Can you work these out from the model? Positions are in its coordinate system, mm. Face numbers are marked on the shaded views. A direction names the side the tool comes from. Round coordinates to 2 decimals unless told otherwise and drop trailing zeros. Loops run counter-clockwise (first coordinate to the right, second up) from the corner with the lowest first, then second, coordinate; pieces in that order, holes last. Notation, with made-up numbers: M -24.5,24.25 L 26.5,24.25 A6 cw 26.5,32.25 Z; hole C 49.25,-27 d6. An arc over 180 degrees is marked long. Answer as CSV lines item,"result".
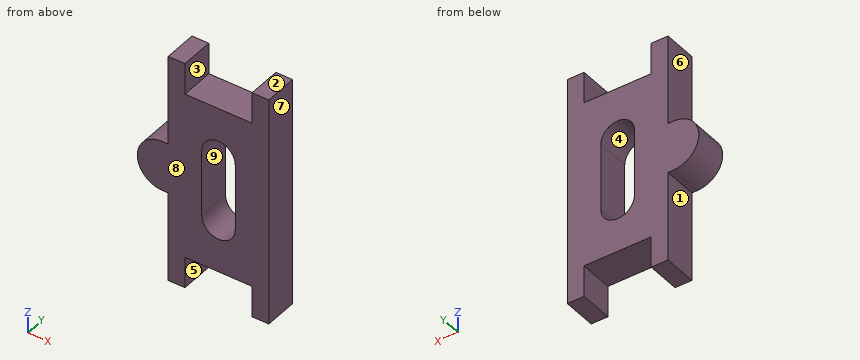
from build123d import *

# Parameters (mm, degrees)
BOSS_EXTRUDE1_DEPTH = 3.175
CUT_EXTRUDE1_REACH  = 5.175


with BuildPart() as part:
    # Sketch2 → Boss-Extrude1 (new body)
    with BuildSketch(Plane(origin=(0, 0, 0), x_dir=(1, 0, 0), z_dir=(0, 1, 0))):
        with BuildLine():
            Line((-3.175, 10.8966), (-3.175, 7.9375))
            Line((-3.175, 7.9375), (3.175, 7.9375))
            Line((3.175, 7.9375), (3.175, 10.8966))
            Line((3.175, 10.8966), (4.7625, 10.8966))
            Line((4.7625, 10.8966), (4.7625, -10.8966))
            Line((4.7625, -10.8966), (3.175, -10.8966))
            Line((3.175, -10.8966), (3.175, -7.9375))
            Line((3.175, -7.9375), (-3.175, -7.9375))
            Line((-3.175, -7.9375), (-3.175, -10.8966))
            Line((-3.175, -10.8966), (-4.7625, -10.8966))
            Line((-4.7625, -10.8966), (-4.7625, -2.38125))
            Line((-4.7625, -2.38125), (-5.30225, -2.38125))
            ThreePointArc((-5.30225, -2.38125), (-7.6835, 0), (-5.30225, 2.38125))
            Line((-5.30225, 2.38125), (-4.7625, 2.38125))
            Line((-4.7625, 2.38125), (-4.7625, 10.8966))
            Line((-4.7625, 10.8966), (-3.175, 10.8966))
        make_face()
    extrude(amount=BOSS_EXTRUDE1_DEPTH)

    # Sketch3 → Cut-Extrude1 (cut, up to next)
    with BuildSketch(Plane(origin=(0, 3.175, 0), x_dir=(1, 0, 0), z_dir=(0, 1, 0)), mode=Mode.PRIVATE) as cut_extrude1_sk1:
        with BuildLine():
            Line((1.5875, 3.175), (1.5875, -3.175))
            ThreePointArc((1.5875, -3.175), (0, -4.7625), (-1.5875, -3.175))
            Line((-1.5875, -3.175), (-1.5875, 3.175))
            ThreePointArc((-1.5875, 3.175), (0, 4.7625), (1.5875, 3.175))
        make_face()
    cut_extrude1_tool1 = extrude(cut_extrude1_sk1.sketch, amount=-CUT_EXTRUDE1_REACH, mode=Mode.PRIVATE) & part.part
    add(cut_extrude1_tool1.solids().sort_by_distance((0, 3.175, 0))[0], mode=Mode.SUBTRACT)


solid = part.part
Item 1: If I drill on line 1 along X through (y, z) = (0.65, 10.25) (1 decimal); line 2 along X through (y, z) = (2.8, -2.5); line 3 along X through (y, z) = (0.75, -5.75), over which ranges is the centre line in solid material (lowest first)? Write a range as from..to.
Output:
line 1,"x = -4.8..-3.2, 3.2..4.8"
line 2,"x = -4.76..-1.59, 1.59..4.76"
line 3,"x = -4.76..4.76"
Item 2: If we section it at C-C on x = 0: Write out the boundary of the cut face in (y, z) (1 decimal).
Output:
outline,"M 0,-7.9 L 3.2,-7.9 L 3.2,-4.8 L 0,-4.8 Z; M 0,4.8 L 3.2,4.8 L 3.2,7.9 L 0,7.9 Z"
Item 3: On a 3-axis mill with a long thin cutter (end or side, diameter ignored), from which of +Z, -Z, +X, -X, +Y, -Y can I reach the whole of each face in a straight line? I mean the marked faces 1, 2, 3, 4 and 5. Say none if no direction works.
Output:
face 1,"-Z, -X, +Y, -Y"
face 2,"+Z, +X, -X, +Y, -Y"
face 3,"+Z, +Y, -Y"
face 4,"+Y, -Y"
face 5,"-Z, +Y, -Y"
Item 4: We'd pull the mould along X, two halves only. Please class the marked faces 6, 7, 8 and 9: released by +X, released by -X, zero draft, split by the parting line, or undercut.
Output:
face 6,"released by -X"
face 7,"released by +X"
face 8,"zero draft"
face 9,"undercut"
Item 5: Will these pins go through, and if not, where does the flat tip stop? pin 1 (1 mm diameter, centred on y = 3, z = 7, fed in from -X); pin 2 (1.6 mm diameter, centred on x = 0, y = 2, fed in from -Z); pin 3 (1 mm diameter, centred on x = -1.5, y = 1.5, fed in from +Z).
Output:
pin 1,"stops at x = -4.76"
pin 2,"stops at z = -7.94"
pin 3,"stops at z = 7.94"
Item 6: If we section it at A-A on z = 0: Write out the boundary of the cut face in (x, y) (1 decimal), then the cut area to 3 significant figures.
Output:
outline,"M -7.7,0 L -1.6,0 L -1.6,3.2 L -7.7,3.2 Z; M 1.6,0 L 4.8,0 L 4.8,3.2 L 1.6,3.2 Z"
area,"29.4 mm2"
Item 7: If we section it at B-B on y = 1.75: Write out the boundary of the cut face in (x, z) (1 decimal), then the cut area to 3 significant figures.
Output:
outline,"M -5.3,-2.4 L -4.8,-2.4 L -4.8,-10.9 L -3.2,-10.9 L -3.2,-7.9 L 3.2,-7.9 L 3.2,-10.9 L 4.8,-10.9 L 4.8,10.9 L 3.2,10.9 L 3.2,7.9 L -3.2,7.9 L -3.2,10.9 L -4.8,10.9 L -4.8,2.4 L -5.3,2.4 A2.4 ccw Z; hole M -1.6,-3.2 A1.6 ccw 1.6,-3.2 L 1.6,3.2 A1.6 ccw -1.6,3.2 Z"
area,"153 mm2"
Item 8: If we section it at D-D on z = -5: Write out the boundary of the cut face in (x, y) (1 decimal).
Output:
outline,"M -4.8,0 L 4.8,0 L 4.8,3.2 L -4.8,3.2 Z"
